Geometry check sheet. Reference: the model listing, model coordinates, mm. A direction names the side the tool comes from. Coordinates: 2 decimals unless noted, no trailing zeros. Use CSV: the item, a comma, the result in double quotes.
```python
from build123d import *

# Parameters (mm, degrees)
F1_DEPTH       = 40
F2_R           = 5
F4_D           = 20
F4_CBORE_D     = 20
F4_CBORE_DEPTH = 20
F5_T           = -2.5


# Not quite as in the source:
# - a shell that OpenCascade refuses in one call is made with other operations: the cavity is built on its own and cut out


with BuildPart() as f1:
    # F0 (on Top) → F1 (new body)
    with BuildSketch(Plane.XY):
        Polygon((29.2738805136, 44.3878389125), (-23.8040558605, 47.5458436484), (-53.0779363741, 3.1580047359), (-29.2738805136, -44.3878389125), (23.8040558605, -47.5458436484), (53.0779363741, -3.1580047359), align=None)
    extrude(amount=F1_DEPTH)

    # F2
    f2_edges = [f1.edges().sort_by_distance(p)[0] for p in [
        (2.734912, 45.966841, 40),
        (41.175908, 20.614917, 40),
        (38.440996, -25.351924, 40),
        (-2.734912, -45.966841, 40),
        (-41.175908, -20.614917, 40),
        (-38.440996, 25.351924, 40),
        (29.273881, 44.387839, 20),
        (-23.804056, 47.545844, 20),
        (-53.077936, 3.158005, 20),
        (-29.273881, -44.387839, 20),
        (23.804056, -47.545844, 20),
        (53.077936, -3.158005, 20),
        (41.175908, 20.614917, 0),
        (38.440996, -25.351924, 0),
        (-2.734912, -45.966841, 0),
        (-41.175908, -20.614917, 0),
        (-38.440996, 25.351924, 0),
        (2.734912, 45.966841, 0),
    ]]
    fillet(f2_edges, radius=F2_R)

    # F4 (through all)
    with Locations(Plane(origin=(-38.4409961173, 25.3519241922, 0), x_dir=(-0.5505527454, -0.83480038, 0), z_dir=(-0.83480038, 0.5505527454, 0))):
        with Locations((1.7491957406, 20)):
            CounterBoreHole(F4_D / 2, F4_CBORE_D / 2, F4_CBORE_DEPTH)

    # F5: a shell. OpenCascade refuses it in one call, so the cavity is built on its own and cut out:
    # the body offset inwards by the wall thickness, plus a prism from it out through each open face.
    f5_core = offset(f1.part, amount=F5_T, mode=Mode.PRIVATE)
    f5_exits = [f5_core.faces().sort_by_distance(p)[0] for p in [
        (0, 0, 2.5),
        (0, 0, 37.5),
    ]]
    add(f5_core, mode=Mode.SUBTRACT)
    extrude(f5_exits, amount=-F5_T, mode=Mode.SUBTRACT)


solid = f1.part
```
1. Release check for a two-part mould opening along Y. For faces 4 (the cylindrical face through (-38.154, -19.473, 36.748)), 5 (the cylindrical face through (-2.32, -44.56, 38.5)), 6 (the cylindrical face through (-52.303, 3.149, 20.21)) record: +Y half, -Y half, draft (parallel to the pull), parting line (faces both ways), or undercut.
The answers:
face 4,"undercut"
face 5,"-Y half"
face 6,"parting line"
2. Section check A-A, the plane z = 13. Count the separate pieces of the cut face and the enclosed holes in it, plus the area to 3 significant figures.
The answers:
separate pieces,"2"
enclosed holes,"2"
area,"1,260 mm^2"
3. Thickness scan on line 1 (Y direction, x = 24, z = 12); line 2 (X direction, y = 4.5, z = 18.5); line 3 (X direction, y = -16.5, z = 19.5). Record the ranges inside material, lowest first. Write a range as [from, to].
The answers:
line 1,"[-46.54, -42.71], [-29.43, -25.11], [-10.74, -6.42], [42.2, 44.7]"
line 2,"[-52.02, -49.2], [-32.54, -27.96], [7.96, 12.54], [46.45, 49.24]"
line 3,"[-43.24, -40.44], [-0.84, 3.7], [39.98, 44.28]"
4. Gauge pin test, flat ends, axial feed: P1, Ø12, axis at x = 34, y = -5, coming from the -Z side; P2, Ø1.5, axis at y = -15, z = 5.5, coming from the -X side; P3, Ø12, axis at y = 37.5, z = 21.5, coming from the -X side. Record the tip position at first contact, or that the pin passes through.
The answers:
P1,"z = 12.91"
P2,"x = -44.36"
P3,"x = -34.21"
5. Set-up check for faces 1 (the flat face through (-2.769, -40.956, 38.732)), 2 (the cylindrical face through (38.154, 19.473, 3.252)), 3 (the cylindrical face through (2.32, 44.56, 1.5)): record each of +Z, -Z, +X, -X, +Y, -Y from which the full face is reachable in a straight line by a thin tool's end or side.
The answers:
face 1,"+Z, -Z"
face 2,"none"
face 3,"-Z, +X, +Y"
